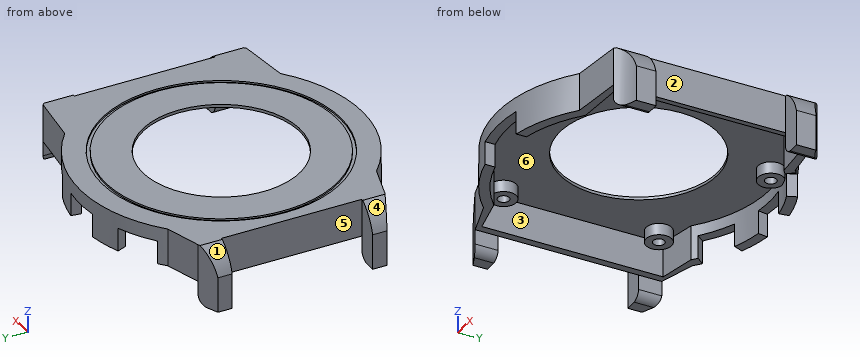
```python
from build123d import *

# Parameters (mm, degrees)
PAD_DEPTH            = 6.5
POCKET_DEPTH         = 6
SKETCH002_R          = 13.5
POCKET001_DEPTH      = 1
SKETCH003_W          = 5.4
SKETCH003_H          = 6.5
PAD001_DEPTH         = 3.5
POCKET002_DEPTH      = 10
SKETCH010_W          = 3.95
SKETCH010_H          = 6.5
PAD002_DEPTH         = 3.5
POCKET005_DEPTH      = 10
SKETCH014_R          = 20.45
SKETCH014_R_2        = 19.85
POCKET008_DEPTH      = 0.3
SKETCH015_R          = 2.2
SKETCH015_R_2        = 0.975
PAD003_DEPTH         = 2
POCKET009_DEPTH      = 4
POCKET010_DEPTH      = 4
PAD004_DEPTH         = 4
POCKET013_DEPTH      = 12.151
POCKET013_DEPTH_BACK = 36.251


with BuildPart() as part:
    # Sketch → Pad (new body)
    with BuildSketch(Plane.XY):
        with BuildLine():
            Line((-22.5019915649, 16), (-22.5019915649, -16))
            Line((-22.5019915649, -16), (-16.2858834578, -17.9))
            ThreePointArc((-16.2858834578, -17.9), (-0.4552796053, -24.1957169863), (15.6009615088, -18.5))
            Line((15.6009615088, -18.5), (24.5395016581, -17.45))
            Line((24.5395016581, 17.45), (24.5395016581, -17.45))
            Line((15.6009615088, 18.5), (24.5395016581, 17.45))
            ThreePointArc((15.6009615088, 18.5), (-0.4552796053, 24.1957169863), (-16.2858834578, 17.9))
            Line((-22.5019915649, 16), (-16.2858834578, 17.9))
        make_face()
    extrude(amount=PAD_DEPTH)

    # Sketch001 → Pocket (cut)
    with BuildSketch(Plane.XY):
        with BuildLine():
            Line((-14.8539557021, 16.9), (-21.2122180433, 15.55))
            Line((-21.2122180433, 15.55), (-21.2122180433, -15.55))
            Line((-21.2122180433, -15.55), (-14.8539557021, -16.9))
            ThreePointArc((-14.8539557021, -16.9), (-0.0760301383, -22.4998715423), (14.739402973, -17))
            Line((14.739402973, -17), (23.6191552218, -16.4))
            Line((23.6191552218, 16.4), (23.6191552218, -16.4))
            Line((14.739402973, 17), (23.6191552218, 16.4))
            ThreePointArc((14.739402973, 17), (-0.0760301383, 22.4998715423), (-14.8539557021, 16.9))
        make_face()
    extrude(amount=POCKET_DEPTH, mode=Mode.SUBTRACT)

    # Sketch002 (on Face19 of Pocket) → Pocket001 (cut)
    with BuildSketch(Plane(origin=(0, 0, 6), x_dir=(1, 0, 0), z_dir=(0, 0, -1))):
        Circle(SKETCH002_R)
    extrude(amount=-POCKET001_DEPTH, mode=Mode.SUBTRACT)

    # Sketch003 (on Face7 of Pad) → Pad001 (join)
    with BuildSketch(Plane.YZ.offset(24.5395016581)):
        with Locations((-14.75, 3.25)):
            Rectangle(SKETCH003_W, SKETCH003_H)
        with Locations((14.75, 3.25)):
            Rectangle(SKETCH003_W, SKETCH003_H)
    extrude(amount=PAD001_DEPTH)

    # Sketch006 (on Face22 of Pad001) → Pocket002 (cut)
    with BuildSketch(Plane.XY.offset(6.5)):
        with BuildLine():
            ThreePointArc((24.5395016581, 17.45), (26.1592830786, 16.2095505764), (28.0395016581, 15.4176006311))
            Line((28.0395016581, 17.45), (28.0395016581, 15.4176006311))
            Line((28.0395016581, 17.45), (24.5395016581, 17.45))
        make_face()
        with BuildLine():
            ThreePointArc((28.0395016581, -15.4176006311), (26.1592830786, -16.2095505765), (24.5395016581, -17.4500000001))
            Line((28.0395016581, -17.45), (24.5395016581, -17.45))
            Line((28.0395016581, -15.4176006311), (28.0395016581, -17.45))
        make_face()
    extrude(amount=-POCKET002_DEPTH, mode=Mode.SUBTRACT)

    # Sketch010 (on Face3 of Pad) → Pad002 (join)
    with BuildSketch(Plane(origin=(-22.5019915649, 0, 0), x_dir=(0, -1, 0), z_dir=(-1, 0, 0))):
        with Locations((-14.025, 3.25)):
            Rectangle(SKETCH010_W, SKETCH010_H)
        with Locations((14.025, 3.25)):
            Rectangle(SKETCH010_W, SKETCH010_H)
    extrude(amount=PAD002_DEPTH)

    # Sketch011 (on Face28 of Pad002) → Pocket005 (cut)
    with BuildSketch(Plane.XY.offset(6.5)):
        Polygon((-26.0019915649, 16), (-22.5019915649, 16), (-26.0019915649, 14.5), align=None)
        Polygon((-22.5019915649, -16), (-26.0019915649, -14.5), (-26.0019915649, -16), align=None)
    extrude(amount=-POCKET005_DEPTH, mode=Mode.SUBTRACT)

    # Sketch014 (on Face10 of Pad) → Pocket008 (cut)
    with BuildSketch(Plane.XY.offset(6.5)):
        Circle(SKETCH014_R)
        Circle(SKETCH014_R_2, mode=Mode.SUBTRACT)
    extrude(amount=-POCKET008_DEPTH, mode=Mode.SUBTRACT)

    # Sketch015 (on Face19 of Pocket) → Pad003 (join)
    with BuildSketch(Plane(origin=(0, 0, 6), x_dir=(1, 0, 0), z_dir=(0, 0, -1))):
        with Locations((-18.42, 13.32)):
            Circle(SKETCH015_R)
        with Locations((-18.42, 13.32)):
            Circle(SKETCH015_R_2, mode=Mode.SUBTRACT)
        with Locations((7.27, 18.56)):
            Circle(SKETCH015_R)
        with Locations((7.27, 18.56)):
            Circle(SKETCH015_R_2, mode=Mode.SUBTRACT)
        with Locations((5.37, -19.79)):
            Circle(SKETCH015_R)
        with Locations((5.37, -19.79)):
            Circle(SKETCH015_R_2, mode=Mode.SUBTRACT)
        with Locations((-18.42, -13.32)):
            Circle(SKETCH015_R)
        with Locations((-18.42, -13.32)):
            Circle(SKETCH015_R_2, mode=Mode.SUBTRACT)
    extrude(amount=PAD003_DEPTH)

    # Sketch016 (on Face4 of Pocket) → Pocket009 (cut)
    with BuildSketch(Plane(origin=(0, 0, 0), x_dir=(1, 0, 0), z_dir=(0, 0, -1))):
        with BuildLine():
            Line((-4.9992330338, 23.6779996848), (-5.0007669662, 21.9372361465))
            ThreePointArc((5.0007669662, 21.9372361465), (0, 22.5), (-5.0007669662, 21.9372361465))
            Line((5.0007669662, 23.6776757675), (5.0007669662, 21.9372361465))
            ThreePointArc((5.0007669662, 23.6776757675), (0.00078388, 24.1999999873), (-4.9992330338, 23.6779996848))
        make_face()
    extrude(amount=-POCKET009_DEPTH, mode=Mode.SUBTRACT)

    # Sketch017 (on Face4 of Pocket) → Pocket010 (cut)
    with BuildSketch(Plane(origin=(0, 0, 0), x_dir=(1, 0, 0), z_dir=(0, 0, -1))):
        with BuildLine():
            ThreePointArc((-3.2541322314, -22.2634369184), (0, -22.5), (3.2541322314, -22.2634369184))
            Line((3.2541322314, -22.2634369184), (3.5, -23.9455632634))
            ThreePointArc((-3.5, -23.9455632634), (0, -24.2), (3.5, -23.9455632634))
            Line((-3.2541322314, -22.2634369184), (-3.5, -23.9455632634))
        make_face()
        with BuildLine():
            ThreePointArc((-13.9498796389, -17.6536358312), (-11.25, -19.4855715851), (-8.3135572795, -20.9077680626))
            Line((-8.3135572795, -20.9077680626), (-8.9416927184, -22.487466094))
            ThreePointArc((-15.0038705449, -18.987466094), (-12.1, -20.9578147716), (-8.9416927184, -22.487466094))
            Line((-13.9498796389, -17.6536358312), (-15.0038705449, -18.987466094))
        make_face()
        with BuildLine():
            ThreePointArc((8.3135572795, -20.9077680626), (11.25, -19.4855715851), (13.9498796389, -17.6536358312))
            Line((13.9498796389, -17.6536358312), (15.0038705449, -18.987466094))
            ThreePointArc((8.9416927184, -22.487466094), (12.1, -20.9578147716), (15.0038705449, -18.987466094))
            Line((8.3135572795, -20.9077680626), (8.9416927184, -22.487466094))
        make_face()
    extrude(amount=-POCKET010_DEPTH, mode=Mode.SUBTRACT)

    # Sketch018 (on Face8 of Pocket005) → Pad004 (join)
    with BuildSketch(Plane(origin=(0, 0, 0), x_dir=(1, 0, 0), z_dir=(0, 0, -1))):
        Polygon((-26.0019915649, 14.5), (-26.0019915649, 12.05), (-22.5019915649, 12.05), (-22.5019915649, 16), align=None)
        Polygon((-26.0019915649, -12.05), (-22.5019915649, -12.05), (-22.5019915649, -16), (-26.0019915649, -14.5), align=None)
        with BuildLine():
            Line((24.5395016581, 17.4500000001), (24.5395016581, 12.05))
            Line((28.0395016581, 12.05), (24.5395016581, 12.05))
            Line((28.0395016581, 15.4176006311), (28.0395016581, 12.05))
            ThreePointArc((24.5395016581, 17.4500000001), (26.1592830786, 16.2095505765), (28.0395016581, 15.4176006311))
        make_face()
        with BuildLine():
            Line((24.5395016581, -12.05), (24.5395016581, -17.45))
            ThreePointArc((28.0395016581, -15.4176006311), (26.1592830786, -16.2095505764), (24.5395016581, -17.45))
            Line((28.0395016581, -12.05), (28.0395016581, -15.4176006311))
            Line((24.5395016581, -12.05), (28.0395016581, -12.05))
        make_face()
    extrude(amount=PAD004_DEPTH)

    # Sketch021 (on Face50 of Pad004) → Pocket013 (cut, two sides)
    with BuildSketch(Plane(origin=(0, -12.05, 0), x_dir=(-1, 0, 0), z_dir=(0, 1, 0))) as pocket013_sk:
        with BuildLine():
            Line((-24.8620157143, 6.5), (-28.0395016581, 6.5))
            Line((-28.0395016581, 6.5), (-28.0395016581, 2.1))
            ThreePointArc((-24.8620157143, 6.5), (-26.8441838951, 4.5841143344), (-28.0395016581, 2.1))
        make_face()
        with BuildLine():
            ThreePointArc((-25.9995016581, -4), (-25.0260575173, -3.5134441408), (-24.5395016581, -2.54))
            Line((-24.5395016581, -4), (-24.5395016581, -2.54))
            Line((-24.5395016581, -4), (-25.9995016581, -4))
        make_face()
        with BuildLine():
            Line((22.5019915649, -4), (22.5019915649, -2.54))
            ThreePointArc((22.5019915649, -2.54), (22.9885474241, -3.5134441408), (23.9619915649, -4))
            Line((22.5019915649, -4), (23.9619915649, -4))
        make_face()
        with BuildLine():
            Line((26.0019915649, 6.5), (26.0019915649, 2.1))
            ThreePointArc((26.0019915649, 2.1), (24.806673802, 4.5841143344), (22.8245056212, 6.5))
            Line((26.0019915649, 6.5), (22.8245056212, 6.5))
        make_face()
    extrude(amount=-POCKET013_DEPTH, mode=Mode.SUBTRACT)
    extrude(pocket013_sk.sketch, amount=POCKET013_DEPTH_BACK, mode=Mode.SUBTRACT)


solid = part.part
```
Verification items for the finished model (mm, model axes). Face numbers are marked on the shaded views. A direction names the side the tool comes from. Round coordinates to 2 decimals unless told otherwise and drop trailing zeros. Order: outer loops, then holes, each group sorted by start corner. A loop starts at its lowest first (then second) coordinate and runs counter-clockwise, first axis right, second up.
1) Cross-section at C-C, the plane x = -2. Record the cut outline in (y, z), plus the area to 3 significant figures.
Geometry says:
outline: (-24.12, 4) - (-22.41, 4) - (-22.41, 6) - (-13.35, 6) - (-13.35, 6.5) - (-19.75, 6.5) - (-19.75, 6.2) - (-20.35, 6.2) - (-20.35, 6.5) - (-24.12, 6.5) - close; (13.35, 6) - (22.41, 6) - (22.41, 4) - (24.12, 4) - (24.12, 6.5) - (20.35, 6.5) - (20.35, 6.2) - (19.75, 6.2) - (19.75, 6.5) - (13.35, 6.5) - close
area: 17.2 mm2
2) Tool access check on the marked faces 4, 5 and 6. Record the directions out of +Z, -Z, +X, -X, +Y, -Y that give a thin tool (end or side, any length) a straight path to the whole face; none if there is none.
Geometry says:
face 4: +Z, -X, +Y, -Y
face 5: +Z, -Z, -X
face 6: -Z
3) Cross-section at B-B, the plane z = -1.5. Record the cut outline in (x, y), plus the area to 3 significant figures.
Geometry says:
outline: (-26, -14.5) - (-22.5, -16) - (-22.5, -12.05) - (-26, -12.05) - close; (-26, 12.05) - (-22.5, 12.05) - (-22.5, 16) - (-26, 14.5) - close; (24.54, -17.45) arc R8.03 cw to (28.04, -15.42) - (28.04, -12.05) - (24.54, -12.05) - close; (24.54, 12.05) - (28.04, 12.05) - (28.04, 15.42) arc R8.03 cw to (24.54, 17.45) - close
area: 51.7 mm2
4) Material ranges on line 1 (Y direction, x = 0, z = 6.4); line 2 (X direction, y = 12, z = 1.75); line 3 (Y direction, x = 7.27, z = 5.1) (3 decimals), recorded low to high.
Geometry says:
line 1: y = -24.2 to -20.45, -19.85 to -13.5, 13.5 to 19.85, 20.45 to 24.2
line 2: x = -22.5 to -21.21, 23.62 to 24.54
line 3: y = -23.082 to -21.293, -20.76 to -19.535, -17.585 to -16.36, 18.681 to 20.899, 21.293 to 23.082
5) Cross-section at A-A, the plane y = 0. Record the cut outline in (x, z), plus the area to 3 significant figures.
Geometry says:
outline: (-22.5, 0) - (-21.21, 0) - (-21.21, 6) - (-13.5, 6) - (-13.5, 6.5) - (-19.85, 6.5) - (-19.85, 6.2) - (-20.45, 6.2) - (-20.45, 6.5) - (-22.5, 6.5) - close; (13.5, 6) - (23.62, 6) - (23.62, 0) - (24.54, 0) - (24.54, 6.5) - (20.45, 6.5) - (20.45, 6.2) - (19.85, 6.2) - (19.85, 6.5) - (13.5, 6.5) - close
area: 22.9 mm2
6) Depth check by flat-ended pin: pin 1 (0.9 mm diameter, centred on x = -7, y = 22, fed in from -Z); pin 2 (12 mm diameter, centred on x = -11, y = -2, fed in from -Z); pin 3 (2 mm diameter, centred on x = 5, y = 20, fed in from -Z). Enter the tip coordinate at first touch or a pass-through.
Geometry says:
pin 1: stops at z = 0
pin 2: stops at z = 6
pin 3: stops at z = 4
7) Draft check along X on the marked faces 1, 2 and 3. Enter one of: +X half, -X half, draft (parallel to the pull), parting line (faces both ways), or undercut.
Geometry says:
face 1: -X half
face 2: +X half
face 3: undercut
